Here's how the part is built. I have some questions about the finished solid (model axes, mm). A direction names the side the tool comes from. Round coordinates to 2 decimals unless told otherwise and drop trailing zeros. Loops run counter-clockwise (first coordinate to the right, second up) from the corner with the lowest first, then second, coordinate; pieces in that order, holes last. Notation, with made-up numbers: (9, -31) -> (66, -31) arc R24 cw to (66, -4) -> close; hole circle Ø4 at (80, -17.75). An arc over 180 degrees is marked (long way). Use one line per item in the form item = value. Start each with the question number.
Item 1: If we section it at C-C (x = 35.5): Write out the boundary of the cut face in (y, z), then the cut area to 3 significant figures.
Item 2: For faces 1 (the face through (26.749, 8.039, -49.963)), 2 (the face through (-17.547, 12.86, -52.874)), 3 (the face through (48, 3, -36)), 4 (the face through (-50.36, 7.19, 24.23)), which set-ups out of +Z, -Z, +X, -X, +Y, -Y let a thin tool reach every point of the face, with its end or its side?
Item 3: If we section it at D-D (z = 4.5): Write out the boundary of the cut face in (x, y).
Item 4: If I drill on L1, parallel to Z at x = -35, y = 1.5; L2, parallel to Z at x = -1.5, y = 14.5; L3, parallel to Y at x = -24, z = 20.5, over which ranges is the centre line in solid material (lowest first)? Write a range as [from, to].
Item 5: If we section it at A-A (y = 12.25): Write out the boundary of the cut face in (x, z).
Item 6: Thinking about a two-plate mould opening in Z: for faces 5 (the face through (52.6, 1.48, 37.69)), 6 (the face through (5.4, 1.5, -46.2)), 7 (the face through (46, 23, -32)), 8 (the face through (-42.28, 1.52, -19.41)), which applies, released by +Z, released by -Z, zero draft, split by the parting line, or undercut?
Item 7: If we section it at B-B (z = 32.5): Write out the boundary of the cut face in (x, y).
Item 8: I'm going to push flat-ended pins straight in: pin 1 Ø6 at (y, z) = (2.5, 23) entering from -X; pin 2 Ø5 at (y, z) = (8.5, -29.5) entering from +X; pin 3 Ø4 at (y, z) = (18.5, 31.5) entering from -X. Where does each tip first touch, or does it pass through?
Autodesk Inventor part; units mm, degrees
ref_plane "YZ Plane" through (0, 0, 0) normal (1, 0, 0) x (0, 1, 0)
ref_plane "XZ Plane" through (0, 0, 0) normal (0, 1, 0) x (-1, 0, 0)
ref_plane "XY Plane" through (0, 0, 0) normal (0, 0, 1) x (1, 0, 0)
sketch "Sketch1" plane through (0, 0, 0) normal (0, 1, 0) x (-1, 0, 0)
  circle A0 centre (0, 0) radius 58.71
  circle A1 centre (0, 0) radius 55.71
  circle A2 centre (0, 0) radius 64.71
  dimension "d0" = 117.42
  dimension "d1" = 3
  dimension "d2" = 6
extrude "Extrusion1" add sketch "Sketch1" along normal blind 23 contours A0
extrude "Extrusion2" add sketch "Sketch1" along normal blind 3 contours A2
sketch "Sketch2" plane through (0, 3, 0) normal (0, 1, 0) x (1, 0, 0)
  circle A0 centre (-4.5, -59.5402) radius 1
  circle A1 centre (0, 0) radius 58.71
  circle A2 centre (0, 0) radius 60.71 construction
  circle A3 centre (4.5, -61.5457) radius 1
  dimension "d7" = 2
  dimension "d8" = 4.5
  dimension "d9" = 4.5
extrude "Extrusion3" cut sketch "Sketch2" against normal up to surface (3 mm away) contours A0 | A3
extrude "Extrusion4" add sketch "Sketch1" along normal blind 3 contours A1
sketch "Sketch3" plane through (0, 0, 0) normal (0, -1, 0) x (1, 0, 0)
  line L0 (64.71, -10) -> (44.71, -10)
  line L1 (44.71, -10) -> (44.71, 10)
  line L2 (44.71, 10) -> (64.71, 10)
  line L3 (64.71, 10) -> (64.71, -10)
  circle A0 centre (0, 0) radius 64.71
  point P0 (64.71, 0)
  point P1 (5.4987, 96.2431)
  point P2 (3.5009, 96.3364)
  dimension "d14" = 20
  dimension "d15" = 20
extrude "Extrusion5" cut sketch "Sketch3" against normal up to surface (23 mm away) contours L0 A0 L3 | L0 L1 L2 A0 | A0 L2 L3 picked at (51.3767, 0)
pattern_circular "Circular Pattern1" count 5 over 360 about axis through (0, -10, 0) along (0, 1, 0) of "Extrusion5"
fillet "Fillet1" radius 3 6 edges at (44.71, 1.5, 10) (44.71, 1.5, -10) (-42.049, 1.5, -18.1897) (-30.2933, 1.5, -34.37) (23.3267, 1.5, -39.4316) (4.3056, 1.5, -45.6119)
properties part number "122mm-CoilForm_3DPrint"
Values found:
q1.outline = (0, -54.1) -> (3, -54.1) -> (3, -46.76) -> (23, -46.76) -> (23, -42.93) -> (3, -42.93) -> (3, 42.93) -> (23, 42.93) -> (23, 46.76) -> (3, 46.76) -> (3, 54.1) -> (0, 54.1) -> close
q1.area = 478 mm2
q2.face_1 = -Z, +Y, -Y
q2.face_2 = +Y
q2.face_3 = -Z, +X, +Y
q2.face_4 = +Y, -Y
q3.outline = (-64.55, 0) -> (44.71, 0) -> (44.71, 3) -> (-55.53, 3) -> (-55.53, 23) -> (-58.54, 23) -> (-58.54, 3) -> (-64.55, 3) -> close
q4.L1 = [-54.43, -37.79], [-27.89, 27.89], [37.79, 54.43]
q4.L2 = [-58.69, -55.69], [55.69, 58.69]
q4.L3 = [0, 3]
q5.outline = (-52.68, -25.91) -> (-50.22, -24.12) arc R55.71 cw to (-50.22, 24.12) -> (-52.68, 25.91) arc R58.71 ccw to start; (-40.93, -42.09) arc R58.71 ccw to (8.37, -58.11) -> (7.43, -55.21) arc R55.71 cw to (-38.46, -40.3) -> close; (-40.93, 42.09) -> (-38.46, 40.3) arc R55.71 cw to (7.43, 55.21) -> (8.37, 58.11) arc R58.71 ccw to start; (26.45, -49.03) -> (27.39, -51.93) arc R58.71 ccw to (57.85, -10) -> (54.81, -10) arc R55.71 cw to start; (26.45, 49.03) arc R55.71 cw to (54.81, 10) -> (57.85, 10) arc R58.71 ccw to (27.39, 51.93) -> close
q6.face_5 = released by +Z
q6.face_6 = undercut
q6.face_7 = zero draft
q6.face_8 = undercut
q7.outline = (-31.65, 0) -> (55.96, 0) -> (55.96, 3) -> (48.89, 3) -> (48.89, 23) -> (45.25, 23) -> (45.25, 3) -> (-31.65, 3) -> close
q8.pin_1 = -61.54
q8.pin_2 = 52.13
q8.pin_3 = 44.51
